Geometry check sheet. Reference: drawing and pictorial views, mm from the part's lowest x, y, z. A direction names the side the tool comes from. Coordinates: 2 decimals unless noted, no trailing zeros. Write each loop counter-clockwise with the first axis right and the second up, starting at its lowest first coordinate (ties: lowest second). Pieces come first, ordered by that corner, then holes. Notation, with made-up numbers: (31.5, -27.75) -> (74.5, -27.75) arc R16 ccw to (74.5, -17.75) -> close; hole circle Ø11 at (14, 42). An arc over 180 degrees is marked (long way). Use a Markdown table: item, result.
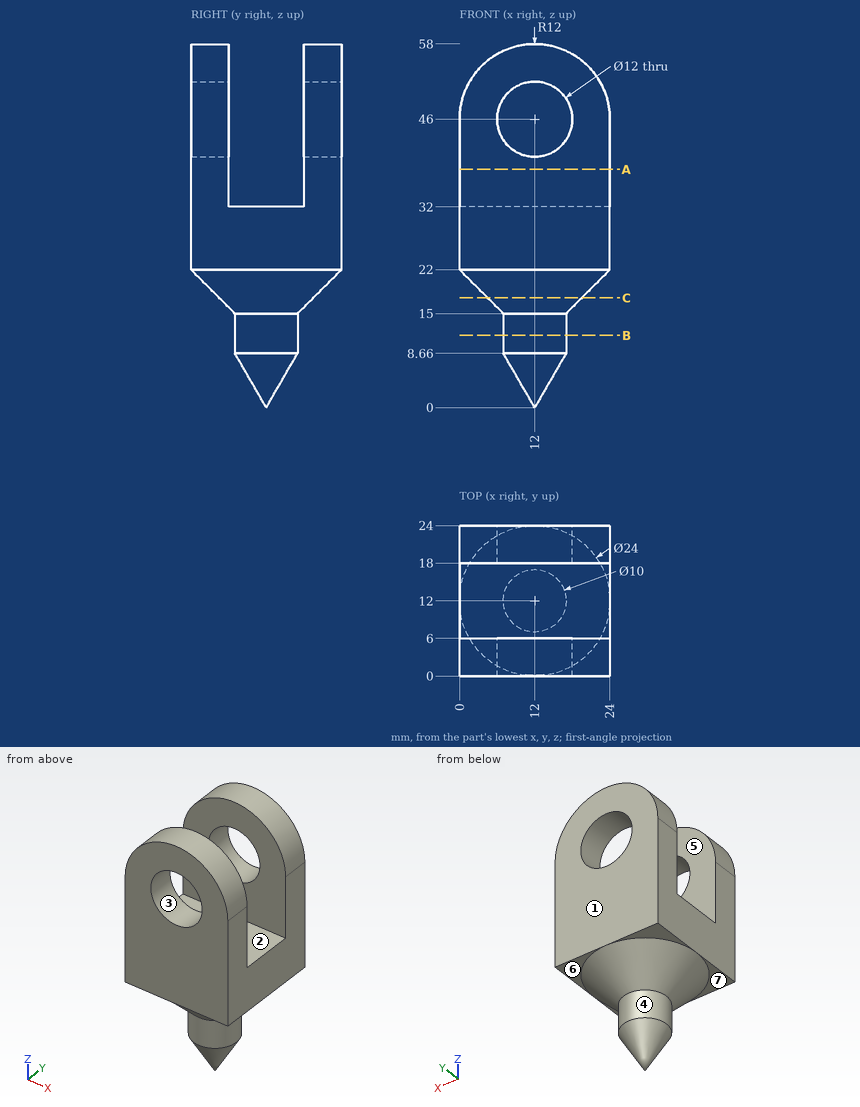
Item 1: Section check C-C on z = 17.5. Record the boundary of the cut face in (x, y).
Answer block:
| item | result |
|---|---|
| outline | circle Ø15 at (12, 12) |
Item 2: Mould release check, pull along Z, two halves, no side actions. Record for the marked faces 1, 2 and 3: +Z half, -Z half, draft (parallel to the pull), parting line (faces both ways), or undercut.
Answer block:
| item | result |
|---|---|
| face 1 | draft |
| face 2 | +Z half |
| face 3 | undercut |
Item 3: Thickness scan on L1, parallel to Y at x = 14.25, z = 35.5; L2, parallel to Z at x = 12, y = 1.75. Record the ranges inside material, lowest first. Write a range as [from, to].
Answer block:
| item | result |
|---|---|
| L1 | y = [0, 6], [18, 24] |
| L2 | z = [20.25, 40], [52, 58] |
Item 4: Tool access check on the marked faces 4, 5, 6 and 7. Record the directions out of +Z, -Z, +X, -X, +Y, -Y that give a thin tool (end or side, any length) a straight path to the whole face; none if there is none.
Answer block:
| item | result |
|---|---|
| face 4 | -Z |
| face 5 | +Z, +X, -X |
| face 6 | -Z, +X, +Y |
| face 7 | -Z, -X, -Y |
Item 5: Section check B-B on z = 11.5. Record the boundary of the cut face in (x, y).
Answer block:
| item | result |
|---|---|
| outline | circle Ø10 at (12, 12) |
Item 6: Depth check by flat-ended pin: P1, Ø9.5, axis at x = 9, y = 3, coming from the -Z side (1 decimal); P2, Ø4, axis at x = 10.5, y = 9, coming from the -Z side (1 decimal); P3, Ø6, axis at x = 5, y = 18.5, coming from the -Z side. Enter the tip coordinate at first touch or a pass-through.
Answer block:
| item | result |
|---|---|
| P1 | stops at z = 8.2 |
| P2 | stops at z = 2.3 |
| P3 | stops at z = 16.55 |
Item 7: Section check A-A on z = 38. Record the boundary of the cut face in (x, y).
Answer block:
| item | result |
|---|---|
| outline | (0, 0) -> (24, 0) -> (24, 6) -> (0, 6) -> close; (0, 18) -> (24, 18) -> (24, 24) -> (0, 24) -> close |
